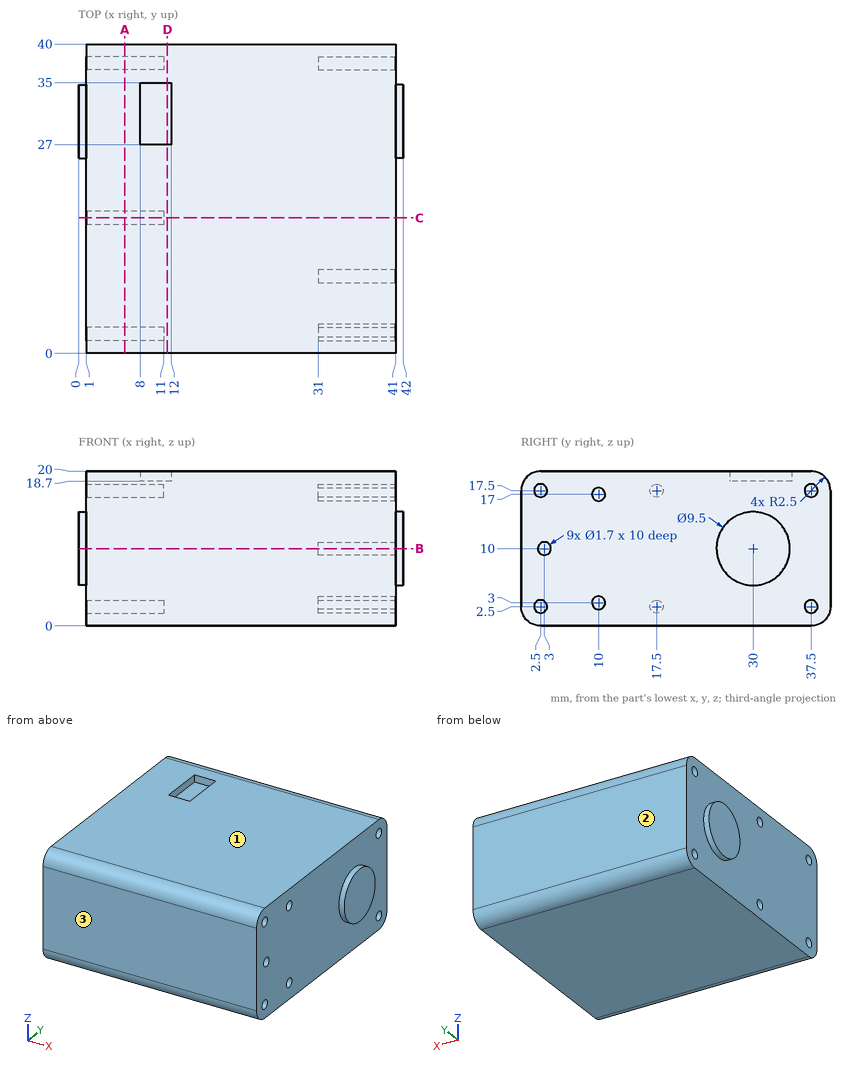
Could you check a few things on this drawing? It's one solid part, dimensions in mm from its lowest x, y, z. Give positions to 0.01 mm unless a question says otherwise; leave off trailing zeros. Order: outer loops, then holes, each group sorted by start corner. A loop starts at its lowest first (then second) coordinate and runs counter-clockwise, first axis right, second up. Notation, with made-up numbers: (-1, 3) - (57, 3) arc R27 cw to (57, 42) - close; hole circle Ø11 at (81, 64). An arc over 180 degrees is marked (long way). One line per question, with ' | ' between items. Start each with the question number.
Item 1: I want a section at B-B on z = 10. Write out the boundary of the cut face in (x, y), then the cut area to 3 significant figures.
Item 2: I want a section at A-A on x = 6. Write out the boundary of the cut face in (y, z), then the cut area to 3 significant figures.
Item 3: I need wall thicknesses on probe 1 along Y at (x, z) = (7.5, 2.5); probe 2 along Y at (x, z) = (37.75, 17.5); probe 3 along Y at (x, z) = (33.5, 10). Which ranges of each line are inside material? Lowest first, please. Write a range as [from, to].
Item 4: I want a section at D-D on x = 11.5. Write out the boundary of the cut face in (y, z).
Item 5: I'm going to push flat-ended pins straight in: pin 1 Ø1.4 at (y, z) = (37.5, 2.5) entering from +X; pin 2 Ø2 at (y, z) = (2.5, 2.5) entering from +X; pin 3 Ø0.7 at (x, z) = (9.5, 19.5) entering from +Y. Where does each tip first touch, or does it pass through?
Item 6: Thinking about a two-plate mould opening in Y: for the marked faces 1, 2 and 3, which applies, pulls with the +Y half, pulls with the -Y half, needs draft (parallel to the pull), parting line crosses it, or undercut?
Item 7: I want a section at C-C on y = 17.5. Write out the boundary of the cut face in (x, z).
Verdict:
1) outline: (0, 25.25) - (1, 25.25) - (1, 0) - (41, 0) - (41, 2.15) - (31, 2.15) - (31, 3.85) - (41, 3.85) - (41, 25.25) - (42, 25.25) - (42, 34.75) - (41, 34.75) - (41, 40) - (1, 40) - (1, 34.75) - (0, 34.75) - close | area: 1,600 mm^2
2) outline: (0, 2.5) arc R2.5 ccw to (2.5, 0) - (37.5, 0) arc R2.5 ccw to (40, 2.5) - (40, 17.5) arc R2.5 ccw to (37.5, 20) - (2.5, 20) arc R2.5 ccw to (0, 17.5) - close; hole circle Ø1.7 at (2.5, 2.5); hole circle Ø1.7 at (2.5, 17.5); hole circle Ø1.7 at (17.5, 2.5); hole circle Ø1.7 at (17.5, 17.5); hole circle Ø1.7 at (37.5, 2.5); hole circle Ø1.7 at (37.5, 17.5) | area: 781 mm^2
3) probe 1: [0, 1.65], [3.35, 16.65], [18.35, 36.65], [38.35, 40] | probe 2: [0, 1.65], [3.35, 9.31], [10.69, 36.65], [38.35, 40] | probe 3: [0, 2.15], [3.85, 40]
4) outline: (0, 2.5) arc R2.5 ccw to (2.5, 0) - (37.5, 0) arc R2.5 ccw to (40, 2.5) - (40, 17.5) arc R2.5 ccw to (37.5, 20) - (35, 20) - (35, 18.7) - (27, 18.7) - (27, 20) - (2.5, 20) arc R2.5 ccw to (0, 17.5) - close
5) pin 1: x = 31 | pin 2: x = 41 | pin 3: y = 39.38
6) face 1: needs draft | face 2: pulls with the +Y half | face 3: pulls with the -Y half
7) outline: (1, 0) - (41, 0) - (41, 20) - (1, 20) - (1, 18.35) - (11, 18.35) - (11, 16.65) - (1, 16.65) - (1, 3.35) - (11, 3.35) - (11, 1.65) - (1, 1.65) - close
